Autodesk Inventor part; units mm, degrees
ref_plane "YZ Plane" through (0, 0, 0) normal (1, 0, 0) x (0, 1, 0)
ref_plane "XZ Plane" through (0, 0, 0) normal (0, 1, 0) x (-1, 0, 0)
ref_plane "XY Plane" through (0, 0, 0) normal (0, 0, 1) x (1, 0, 0)
sketch "Sketch1" plane through (0, 0, 0) normal (0, 0, 1) x (1, 0, 0)
  line L0 (-22.189, 41.743) -> (-4.409, 41.743)
  line L1 (-4.409, 41.743) -> (-4.409, 23.963)
  line L2 (-4.409, 23.963) -> (-22.189, 23.963)
  line L3 (-22.189, 23.963) -> (-22.189, 41.743)
  point P0 (0, 0)
  dimension "d0" = 17.78
  dimension "d1" = 17.78
extrude "Plate1" add sketch "Sketch1" along normal blind 1.27
sketch "Sketch2" plane through (-4.409, 40.473, 1.27) normal (0, 1, 0) x (-1, 0, 0)
  line L0 (17.78, 0) -> (0, 0)
  line L1 (0, 0) -> (0, -30)
  line L2 (0, -30) -> (17.78, -30)
  line L3 (17.78, -30) -> (17.78, 0)
edge flange "Flange1" height 30 angle 90 thickness 1.27 bend radius 1.27 thickness toward (0, 1, 0) relief straight relief width 1.27 relief depth 0.635 edges at (-13.299, 41.743, 0) wall of the first edge with corners at (-22.189, 40.473, 1.27) (-4.409, 40.473, 1.27) (-4.409, 40.473, -28.73) (-22.189, 40.473, -28.73)
bend "Bend1"
corner "Corner1"
sketch "Sketch4" plane through (-22.189, 41.743, -28.73) normal (0, 1, 0) x (1, 0, 0)
  circle A0 centre (12.7, -10.95) radius 2
  circle A1 centre (5.08, -10.95) radius 2
  line L0 (17.78, 0) -> (17.78, -27.46)
  line L1 (0, -27.46) -> (0, 0)
  line L2 (0, -27.46) -> (17.78, -27.46)
  point P0 (22.189, -28.73)
  dimension "d26" = 4
  dimension "d27" = 4
  dimension "d29" = 5.08
  dimension "d30" = 5.08
  dimension "d31" = 16.51
  dimension "d32" = 16.51
extrude "Extrusion2" cut sketch "Sketch4" against normal blind 2.54
sketch "Sketch5" plane through (-4.409, 25.233, 0) normal (0, -1, 0) x (1, 0, 0)
  line L0 (-17.78, 0) -> (0, 0)
  line L1 (0, 0) -> (0, 50.8)
  line L2 (0, 50.8) -> (-17.78, 50.8)
  line L3 (-17.78, 50.8) -> (-17.78, 0)
edge flange "Flange2" height 50.8 angle 90 thickness 1.27 bend radius 1.27 thickness toward (0, -1, 0) relief straight relief width 1.27 relief depth 0.635 edges at (-13.299, 23.963, 1.27) wall of the first edge with corners at (-22.189, 25.233, 0) (-4.409, 25.233, 0) (-4.409, 25.233, 50.8) (-22.189, 25.233, 50.8)
bend "Bend2"
corner "Corner2"
sketch "Sketch6" plane through (-4.409, 23.963, 49.53) normal (0, 0, 1) x (1, 0, 0)
  line L0 (-17.78, 0) -> (0, 0)
  line L1 (0, 0) -> (0, 15.24)
  line L2 (0, 15.24) -> (-17.78, 15.24)
  line L3 (-17.78, 15.24) -> (-17.78, 0)
edge flange "Flange3" height 15.24 angle 90 thickness 1.27 bend radius 1.27 thickness toward (0, 0, 1) relief straight relief width 1.27 relief depth 0.635 edges at (-13.299, 25.233, 50.8) wall of the first edge with corners at (-22.189, 23.963, 49.53) (-4.409, 23.963, 49.53) (-4.409, 39.203, 49.53) (-22.189, 39.203, 49.53)
bend "Bend3"
corner "Corner3"
sketch "Sketch7" plane through (-22.189, 40.473, 52.07) normal (0, 1, 0) x (-1, 0, 0)
  line L0 (-17.78, 0) -> (0, 0)
  line L1 (0, 0) -> (0, 27.46)
  line L2 (0, 27.46) -> (-17.78, 27.46)
  line L3 (-17.78, 27.46) -> (-17.78, 0)
edge flange "Flange4" height 30 angle 90 thickness 1.27 bend radius 1.27 thickness toward (0, 1, 0) relief straight relief width 1.27 relief depth 0.635 edges at (-13.299, 39.203, 50.8) wall of the first edge with corners at (-4.409, 40.473, 52.07) (-22.189, 40.473, 52.07) (-22.189, 40.473, 79.53) (-4.409, 40.473, 79.53)
bend "Bend4"
corner "Corner4"
sketch "Sketch9" plane through (-22.189, 41.743, 79.53) normal (0, 1, 0) x (1, 0, 0)
  circle A0 centre (5.08, 10.95) radius 1.9939
  circle A1 centre (12.7, 10.95) radius 1.9939
  line L0 (0, 0) -> (0, 27.46)
  line L1 (17.78, 27.46) -> (17.78, 0)
  point P0 (22.189, 79.53)
  dimension "d69" = 3.9878
  dimension "d70" = 3.9878
  dimension "d71" = 5.08
  dimension "d73" = 16.51
  dimension "d74" = 16.51
  dimension "d79" = 7.62
extrude "Extrusion4" cut sketch "Sketch9" against normal blind 5.08
sketch "Sketch10" plane through (-22.189, 25.233, 2.54) normal (0, 1, 0) x (1, 0, 0)
  point P0 (22.189, 2.54)
equation "\"d3\" = BendReliefWidth"
equation "\"d4\" = BendReliefDepth"
equation "\"d5\" = MinimumRemnant"
equation "\"d6\" = BendRadius"
equation "\"d9\" = BendRadius"
equation "\"d10\" = CornerReliefSize"
equation "\"d11\" = GapSize"
equation "\"d12\" = JacobiRadiusSize"
equation "\"d35\" = BendReliefWidth"
equation "\"d36\" = BendReliefDepth"
equation "\"d37\" = MinimumRemnant"
equation "\"d38\" = BendRadius"
equation "\"d41\" = BendRadius"
equation "\"d42\" = CornerReliefSize"
equation "\"d43\" = GapSize"
equation "\"d44\" = JacobiRadiusSize"
equation "\"d45\" = BendReliefWidth"
equation "\"d46\" = BendReliefDepth"
equation "\"d47\" = MinimumRemnant"
equation "\"d48\" = BendRadius"
equation "\"d51\" = BendRadius"
equation "\"d52\" = CornerReliefSize"
equation "\"d53\" = GapSize"
equation "\"d54\" = JacobiRadiusSize"
equation "\"d55\" = BendReliefWidth"
equation "\"d56\" = BendReliefDepth"
equation "\"d57\" = MinimumRemnant"
equation "\"d58\" = BendRadius"
equation "\"d61\" = BendRadius"
equation "\"d62\" = CornerReliefSize"
equation "\"d63\" = GapSize"
equation "\"d64\" = JacobiRadiusSize"
equation "\"BendRadius\" = Thickness"
equation "\"BendReliefWidth\" = Thickness"
equation "\"BendReliefDepth\" = 0.5 * Thickness"
equation "\"CornerReliefSize\" = 4 * Thickness"
equation "\"MinimumRemnant\" = 2 * Thickness"
equation "\"TransitionRadius\" = BendRadius"
equation "\"JacobiRadiusSize\" = Thickness"
equation "\"GapSize\" = Thickness"
equation "\"d2\" = BendRadius"
properties part number "Hew battery holder"
The listing builds one solid part. Answer for the finished solid, in the listing's coordinates (mm). A direction names the side the tool comes from. Round coordinates to 2 decimals unless told otherwise and drop trailing zeros. Write each loop counter-clockwise with the first axis right and the second up, starting at its lowest first coordinate (ties: lowest second). Pieces come first, ordered by that corner, then holes. Notation, with made-up numbers: (78, 63.5) -> (103, 63.5) arc R27 ccw to (103, 84.5) -> close; hole circle Ø10 at (-29.5, -13.75). An arc over 180 degrees is marked (long way). Use CSV: the item, a comma, the result in double quotes. Start each with the question number.
(1) Section C-C on x = -18 is taken. Give the vertices of the cut face in (y, z).
(2) Section D-D on x = -13.5 is taken. Give the vertices of the cut face in (y, z).
(3) The mould has two halves that part along X. Classify faces 1 (the face through (-15.2, 41.12, -18.38)), 2 (the face through (-13.17, 24.73, 50.08)), 3 (the face through (-4.409, 25, 34)): released by +X, released by -X, zero draft, split by the parting line, or undercut.
(4) Which of the six approach directions +Z, -Z, +X, -X, +Y, -Y give full straight-line access (tool end or side, diameter ignored) to faces 4 (the face through (-13, 40.473, -15)), 5 (the face through (-13, 40.473, 66)), 6 (the face through (-13, 33, 1.27))?
(5) Section B-B on z = 68.58 is taken. Give the vertices of the cut face in (x, y), then the cut area to 3 significant figures.
(6) Consider L1, parallel to X at y = 41, z = 68.58; L2, parallel to Z at x = -13.75, y = 38.5; L3, parallel to Y at x = -14.75, z = -9.5. Determine where each line is inside the solid, lowest interval first. Write a range as from..to.
(7) Each of these flat-tipped pins is pushed along its axis until it touches: pin 1 (9 mm diameter, centred on x = -14, z = 59.5, fed in from -Y); pin 2 (4 mm diameter, centred on x = -12, y = 30.5, fed in from -Z); pin 3 (10 mm diameter, centred on x = -12.5, y = 29.5, fed in from +Z); pin 4 (5 mm diameter, centred on y = 26, z = 37, fed in from +X). Where does it stop, or does it pass through?
(8) Section A-A on y = 30 is taken. Give the vertices of the cut face in (x, z).
A:
1,outline,"(23.96, 2.54) arc R2.54 ccw to (26.5, 0) -> (39.2, 0) arc R1.27 cw to (40.47, -1.27) -> (40.47, -15.99) -> (41.74, -15.99) -> (41.74, -1.27) arc R2.54 ccw to (39.2, 1.27) -> (26.5, 1.27) arc R1.27 cw to (25.23, 2.54) -> (25.23, 48.26) arc R1.27 cw to (26.5, 49.53) -> (39.2, 49.53) arc R2.54 ccw to (41.74, 52.07) -> (41.74, 66.8) -> (40.47, 66.8) -> (40.47, 52.07) arc R1.27 cw to (39.2, 50.8) -> (26.5, 50.8) arc R2.54 ccw to (23.96, 48.26) -> close; (40.47, -28.73) -> (41.74, -28.73) -> (41.74, -19.57) -> (40.47, -19.57) -> close; (40.47, 70.36) -> (41.74, 70.36) -> (41.74, 79.53) -> (40.47, 79.53) -> close"
2,outline,"(23.96, 2.54) arc R2.54 ccw to (26.5, 0) -> (39.2, 0) arc R1.27 cw to (40.47, -1.27) -> (40.47, -28.73) -> (41.74, -28.73) -> (41.74, -1.27) arc R2.54 ccw to (39.2, 1.27) -> (26.5, 1.27) arc R1.27 cw to (25.23, 2.54) -> (25.23, 48.26) arc R1.27 cw to (26.5, 49.53) -> (39.2, 49.53) arc R2.54 ccw to (41.74, 52.07) -> (41.74, 79.53) -> (40.47, 79.53) -> (40.47, 52.07) arc R1.27 cw to (39.2, 50.8) -> (26.5, 50.8) arc R2.54 ccw to (23.96, 48.26) -> close"
3,face 1,"undercut"
3,face 2,"zero draft"
3,face 3,"released by +X"
4,face 4,"-Z, +X, -X, -Y"
4,face 5,"+Z, +X, -X, -Y"
4,face 6,"+X, -X, +Y"
5,outline,"(-22.19, 40.47) -> (-19.1, 40.47) -> (-19.1, 41.74) -> (-22.19, 41.74) -> close; (-15.12, 40.47) -> (-11.48, 40.47) -> (-11.48, 41.74) -> (-15.12, 41.74) -> close; (-7.5, 40.47) -> (-4.41, 40.47) -> (-4.41, 41.74) -> (-7.5, 41.74) -> close"
5,area,"12.5 mm²"
6,L1,"x = -22.19..-19.1, -15.12..-11.48, -7.5..-4.41"
6,L2,"z = 0..1.27, 49.53..50.8"
6,L3,"y = 40.47..41.74"
7,pin 1,"stops at y = 40.47"
7,pin 2,"stops at z = 0"
7,pin 3,"stops at z = 50.8"
7,pin 4,"stops at x = -4.41"
8,outline,"(-22.19, 0) -> (-4.41, 0) -> (-4.41, 1.27) -> (-22.19, 1.27) -> close; (-22.19, 49.53) -> (-4.41, 49.53) -> (-4.41, 50.8) -> (-22.19, 50.8) -> close"
